Build history of the part. All positions in model axes, mm. A direction names the side the tool comes from. Round coordinates to 2 decimals unless told otherwise and drop trailing zeros. Write each loop counter-clockwise with the first axis right and the second up, starting at its lowest first coordinate (ties: lowest second). Pieces come first, ordered by that corner, then holes. Notation, with made-up numbers: (-20.75, -29.75) -> (15.25, -29.75) arc R16 ccw to (15.25, -11.75) -> close; hole circle Ø9 at (10.25, -17). An arc over 180 degrees is marked (long way). Answer in a Markdown table with one row per item. Add a question column.
from build123d import *

# Parameters (mm, degrees)
BOSS_EXTRUDE1_DEPTH = 45
CUT_EXTRUDE1_DEPTH  = 126
SKETCH3_W           = 26
SKETCH3_H           = 15
CUT_EXTRUDE2_DEPTH  = 81.932070281
BOSS_EXTRUDE2_DEPTH = 25
SKETCH5_R           = 15
CUT_EXTRUDE3_DEPTH  = 102.734949747


with BuildPart() as part:
    # Sketch1 → Boss-Extrude1 (new body)
    with BuildSketch(Plane.XY):
        Polygon((-50, 0), (-50, 60), (-35, 60), (-35, 15), (35, 15), (35, 60), (50, 60), (50, 0), align=None)
    extrude(amount=BOSS_EXTRUDE1_DEPTH)

    # Sketch2 → Cut-Extrude1 (cut, through all)
    with BuildSketch(Plane(origin=(50, 0, 0), x_dir=(0, 0, -1), z_dir=(1, 0, 0))):
        Polygon((-15, 60), (-45, 60), (-45, 28), align=None)
    extrude(amount=-CUT_EXTRUDE1_DEPTH, mode=Mode.SUBTRACT)

    # Sketch3 → Cut-Extrude2 (cut, through all)
    with BuildSketch(Plane(origin=(0, 15, 0), x_dir=(1, 0, 0), z_dir=(0, 1, 0))):
        with Locations((0, -37.5)):
            Rectangle(SKETCH3_W, SKETCH3_H)
    extrude(amount=-CUT_EXTRUDE2_DEPTH, mode=Mode.SUBTRACT)

    # Sketch4 → Boss-Extrude2 (add)
    with BuildSketch(Plane(origin=(0, 0, 0), x_dir=(-1, 0, 0), z_dir=(0, 0, -1))):
        with BuildLine():
            Line((25, 15), (25, 60))
            ThreePointArc((25, 60), (0, 85), (-25, 60))
            Line((-25, 60), (-25, 15))
            Line((-25, 15), (25, 15))
        make_face()
    extrude(amount=-BOSS_EXTRUDE2_DEPTH)

    # Sketch5 → Cut-Extrude3 (cut, through all)
    with BuildSketch(Plane.XY.offset(25)):
        with Locations((0, 60)):
            Circle(SKETCH5_R)
    extrude(amount=-CUT_EXTRUDE3_DEPTH, mode=Mode.SUBTRACT)


solid = part.part
(1) Probe line 1 along X through (y, z) = (29, 5); line 2 along Y through (x, z) = (0, 14.5); line 3 along Z through (x, y) = (6, 38.5). List the from-to ranges inside material, lowest first.
(2) Drop flat-ended pins along their axis: P1, Ø8, axis at x = -31.5, z = 36, coming from the +Y side; P2, Ø10, axis at x = 3, z = 33.5, coming from the +Y side; P3, Ø25, axis at x = -2.5, y = 63, coming from the +Z side. Give the stop position or say it passes through.
(3) Saw through at C-C (x = 0). List the corners of the cut face in (y, z), plus the area to 3 significant figures.
(4) Saw through at A-A (z = 37.5). List the corners of the cut face in (x, y).
(5) Mould opens along Y. For faces 6 (the face through (-50, 23, 22)), 7 (the face through (-3.252, 45.357, 12.675)), 8 (the face through (-0.55, 84.994, 12.325)) say: pulls with the +Y half, pulls with the -Y half, needs draft (parallel to the pull), parting line crosses it, or undercut.
(6) Saw through at D-D (y = 55). List the corners of the cut face in (x, z), plus the area to 3 significant figures.
(7) Which spindle directions (+Z, -Z, +X, -X, +Y, -Y) get a long thin tool onto all of the face, cutting with end or side? Do faces 1 (the face through (35, 32, 17)), 2 (the face through (43, 44, 30)), 3 (the face through (42, 60, 7)), 4 (the face through (0, 43, 25)), 5 (the face through (-13, 8, 38)). Say none if no direction does.
(8) Saw through at B-B (y = 23). List the corners of the cut face in (x, z), plus the area to 3 significant figures.
Answer sheet:
| question | item | result |
|---|---|---|
| 1 | line 1 | x = -50 to -35, -25 to 25, 35 to 50 |
| 1 | line 2 | y = 0 to 45, 75 to 85 |
| 1 | line 3 | z = 0 to 25 |
| 2 | P1 | stops at y = 39.67 |
| 2 | P2 | stops at y = 15 |
| 2 | P3 | stops at z = 25 |
| 3 | outline | (0, 0) -> (45, 0) -> (45, 25) -> (15, 25) -> (15, 30) -> (0, 30) -> close; (75, 0) -> (85, 0) -> (85, 25) -> (75, 25) -> close |
| 3 | area | 1,450 mm² |
| 4 | outline | (-50, 0) -> (-13, 0) -> (-13, 15) -> (-35, 15) -> (-35, 36) -> (-50, 36) -> close; (13, 0) -> (50, 0) -> (50, 36) -> (35, 36) -> (35, 15) -> (13, 15) -> close |
| 5 | face 6 | needs draft |
| 5 | face 7 | undercut |
| 5 | face 8 | pulls with the +Y half |
| 6 | outline | (-50, 0) -> (-35, 0) -> (-35, 19.69) -> (-50, 19.69) -> close; (-25, 0) -> (-14.14, 0) -> (-14.14, 25) -> (-25, 25) -> close; (14.14, 0) -> (25, 0) -> (25, 25) -> (14.14, 25) -> close; (35, 0) -> (50, 0) -> (50, 19.69) -> (35, 19.69) -> close |
| 6 | area | 1,130 mm² |
| 7 | face 1 | +Z, -Z, +Y |
| 7 | face 2 | +Z, +X, +Y |
| 7 | face 3 | +Z, -Z, +X, +Y |
| 7 | face 4 | +Z, +Y |
| 7 | face 5 | +Z, +Y, -Y |
| 8 | outline | (-50, 0) -> (-35, 0) -> (-35, 45) -> (-50, 45) -> close; (-25, 0) -> (25, 0) -> (25, 25) -> (-25, 25) -> close; (35, 0) -> (50, 0) -> (50, 45) -> (35, 45) -> close |
| 8 | area | 2,600 mm² |
